Source: three-view drawing plus pictorial views. Frame: mm from the lowest corner of the part. Give positions to 0.01 mm unless a question says otherwise; leave off trailing zeros. Order: outer loops, then holes, each group sorted by start corner. A loop starts at its lowest first (then second) coordinate and runs counter-clockwise, first axis right, second up.
1) Section C-C, the plane x = 35. Return loops of the section in (y, z) (3 decimals), plus the area to 3 significant figures.
2) First-contact query: P1, Ø1.9, axis at x = 5, z = 15, coming from the +Y side. Flat tip, straight axial feed; report the tip coordinate or a pass-through.
3) Section A-A, the plane z = 5. Return loops of the section in (x, y) (3 decimals).
4) Section B-B, the plane y = 1.55. Give the number of separate pieces and of enclosed holes in the cut face, plus the area to 3 significant figures.
5) Material intervals for line 1 (Z direction, x = 25, y = 0.7); line 2 (Z direction, x = 24, y = 1.15); line 3 (X direction, y = 2.2, z = 35.5), sorted ascending.
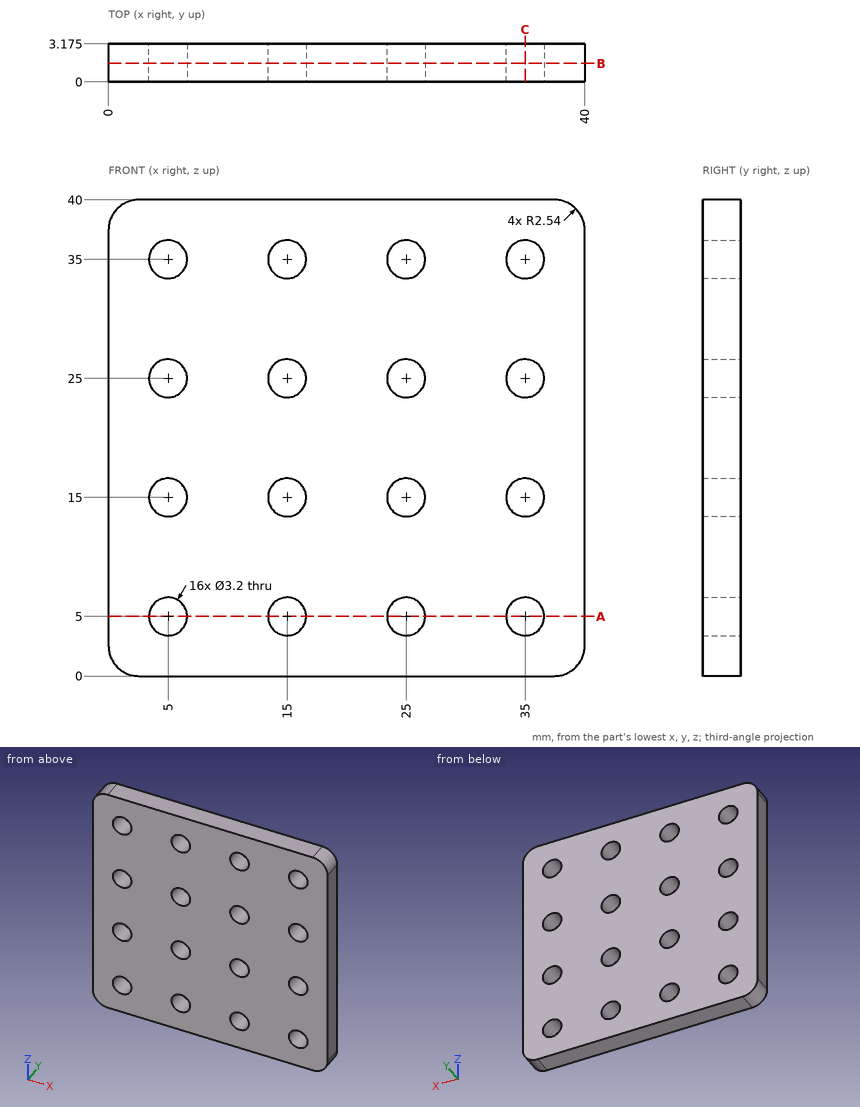
From the geometry:
1. outline: (0, 0) - (3.175, 0) - (3.175, 3.4) - (0, 3.4) - close; (0, 6.6) - (3.175, 6.6) - (3.175, 13.4) - (0, 13.4) - close; (0, 16.6) - (3.175, 16.6) - (3.175, 23.4) - (0, 23.4) - close; (0, 26.6) - (3.175, 26.6) - (3.175, 33.4) - (0, 33.4) - close; (0, 36.6) - (3.175, 36.6) - (3.175, 40) - (0, 40) - close
1. area: 86.4 mm2
2. P1: passes through
3. outline: (0, 0) - (3.4, 0) - (3.4, 3.175) - (0, 3.175) - close; (6.6, 0) - (13.4, 0) - (13.4, 3.175) - (6.6, 3.175) - close; (16.6, 0) - (23.4, 0) - (23.4, 3.175) - (16.6, 3.175) - close; (26.6, 0) - (33.4, 0) - (33.4, 3.175) - (26.6, 3.175) - close; (36.6, 0) - (40, 0) - (40, 3.175) - (36.6, 3.175) - close
4. separate pieces: 1
4. enclosed holes: 16
4. area: 1,470 mm2
5. line 1: z = 0 to 3.4, 6.6 to 13.4, 16.6 to 23.4, 26.6 to 33.4, 36.6 to 40
5. line 2: z = 0 to 3.75, 6.25 to 13.75, 16.25 to 23.75, 26.25 to 33.75, 36.25 to 40
5. line 3: x = 0 to 3.48, 6.52 to 13.48, 16.52 to 23.48, 26.52 to 33.48, 36.52 to 40
